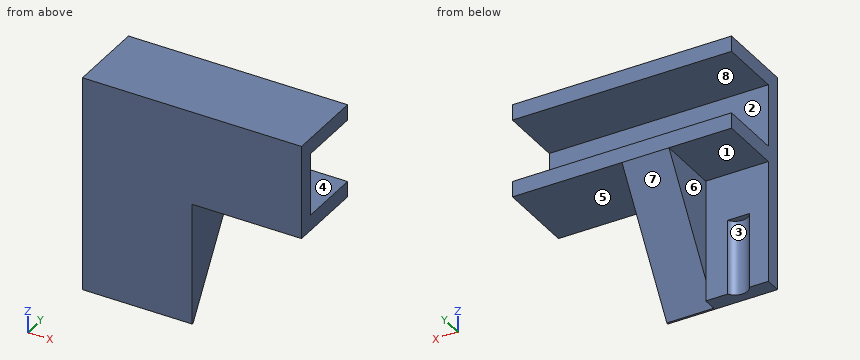
Autodesk Inventor part; units mm, degrees
ref_plane "YZ Plane" through (0, 0, 0) normal (1, 0, 0) x (0, 1, 0)
ref_plane "XZ Plane" through (0, 0, 0) normal (0, 1, 0) x (-1, 0, 0)
ref_plane "XY Plane" through (0, 0, 0) normal (0, 0, 1) x (1, 0, 0)
sketch "Sketch1" plane through (0, 0, 0) normal (0, 1, 0) x (-1, 0, 0)
  line L0 (70, 80) -> (0, 80)
  line L1 (0, 80) -> (0, 0)
  line L2 (0, 0) -> (70, 0)
  line L3 (70, 0) -> (70, 80)
  line L4 (0, 0) -> (30, 0)
  line L5 (30, 0) -> (30, 60)
  line L6 (30, 60) -> (0, 60)
  line L7 (0, 60) -> (0, 0)
  point P0 (0, 60)
  dimension "d0" = 80
  dimension "d1" = 70
  dimension "d2" = 30
  dimension "d3" = 60
extrude "Extrusion1" add sketch "Sketch1" along normal blind 10 contours L3 L2 L5 L6 L1 L0
sketch "Sketch2" plane through (0, 0, 80) normal (1, 0, 0) x (0, 0, -1)
  line L0 (0, 0) -> (20, 0) construction
  line L1 (0, 10) -> (20, 10) construction
  line L2 (0, 0) -> (0, 10) construction
  line L3 (-50, 0) -> (0, 0)
  line L4 (0, 0) -> (0, 50)
  line L5 (0, 50) -> (-10, 50)
  line L6 (-10, 50) -> (-10, 10)
  line L7 (-10, 10) -> (-50, 10)
  line L8 (-50, 10) -> (-50, 0)
  point P0 (80, 0)
  dimension "d6" = 50
  dimension "d7" = 50
  dimension "d8" = 40
  dimension "d9" = 40
extrude "Extrusion2" add sketch "Sketch2" along normal mid plane 140
sketch "Sketch4" plane through (-30, 0, 0) normal (0, 0, -1) x (-1, 0, 0)
  circle A0 centre (21, 14) radius 8.0623
  point P0 (-30, 0)
extrude "Extrusion3" cut sketch "Sketch4" against normal blind 50
sketch "Sketch6" plane through (-30, 0, 60) normal (1, 0, 0) x (0, 0, -1)
  line L0 (-20, 50) -> (-20, 10) construction
  line L1 (60, 0) -> (-20, 50)
  line L2 (-20, 50) -> (-20, 0)
  line L3 (-20, 0) -> (60, 0)
extrude "Extrusion4" add sketch "Sketch6" along normal blind 30
sketch "Sketch7" plane through (-70, 0, 0) normal (-1, 0, 0) x (0, 0, 1)
  line L0 (2, 52) -> (-22, 52)
  line L1 (-22, 52) -> (-22, -1)
  line L2 (-22, -1) -> (2, -1)
  line L3 (2, -1) -> (2, 52)
extrude "Extrusion5" cut sketch "Sketch7" against normal blind 1000
sketch "Sketch8" plane through (-70, 0, 2) normal (-1, 0, 0) x (0, 0, 1)
  line L0 (128, 0) -> (138, 0)
  line L1 (138, 0) -> (138, 50)
  line L2 (138, 50) -> (128, 50)
  line L3 (128, 50) -> (128, 0)
  point P0 (-2, 0)
  dimension "d18" = 10
extrude "Extrusion6" add sketch "Sketch8" against normal up to surface (140 mm away)
properties part number "GiroMotorKrepl"
Design review of the part built by this model. Coordinates are the model's own, in mm. Face numbers are marked on the shaded views. A direction names the side the tool comes from. Round coordinates to 2 decimals unless told otherwise and drop trailing zeros. Write each loop counter-clockwise with the first axis right and the second up, starting at its lowest first coordinate (ties: lowest second). Pieces come first, ordered by that corner, then holes. Notation, with made-up numbers: (47.25, 47) - (95.25, 47) arc R25 ccw to (95.25, 71) - close; hole circle Ø11 at (32, 38). An arc over 180 degrees is marked (long way). Return JSON: item names as keys, results as strings. Group by question number.
Item 1: Machinability: for the marked faces 5, 6, 7 and 8, which of the approach directions +Z, -Z, +X, -X, +Y, -Y give a long, thin tool a straight path to every point of the face, cutting with its end or side? Answer none if there is none.
Item 2: We need section A-A on y = 32.5. Write out the cut boundary in (x, z).
Item 3: Insertion check: P1, Ø25, axis at x = 37, y = 20, coming from the -Z side; P2, Ø12, axis at x = 52.5, z = 122.5, coming from the +Y side; P3, Ø2.5, axis at y = 5, z = 6.5, coming from the +X side. Each pin has a flat end and moves straight along its axis. Give the tip position at first contact, or say it passes through.
Item 4: For probe 1 along Z at (x, y) = (-35.5, 46); probe 2 along X at (y, z) = (24, 41); probe 3 along Y at (x, z) = (-43, 18.5), list the stretches that pass through material, from the lowest coordinate up. Write a range as [from, to].
Item 5: We need section D-D on y = 14. Write out the cut boundary in (x, z).
Item 6: We need section C-C on z = 24. Write out the cut boundary in (x, y), and give its area (3 significant figures).
Item 7: We need section B-B on x = -22.5. Write out the cut boundary in (y, z).
Item 8: The part is to be moulded in two halves that separate along Z. For the marked faces 1, 2, 3 and 4, say which applies: pulls with the +Z half, pulls with the -Z half, needs draft (parallel to the pull), parting line crosses it, or undercut.
Model answer:
{
 "1": {"face 5": "-Z, +X, +Y, -Y", "face 6": "-Z, -X, +Y", "face 7": "-Z, +X, +Y", "face 8": "+X, -X, +Y"},
 "2": {"outline": "(-70, 80) - (-30, 80) - (-30, 52) - (0, 52) - (0, 80) - (70, 80) - (70, 90) - (-70, 90) - close; (-70, 130) - (70, 130) - (70, 140) - (-70, 140) - close"},
 "3": {"P1": "stops at z = 80", "P2": "stops at y = 10", "P3": "stops at x = 0"},
 "4": {"probe 1": "z = [80, 90], [130, 140]", "probe 2": "x = [-30, 0]", "probe 3": "y = [0, 10]"},
 "5": {"outline": "(-70, 80) - (-30, 80) - (-30, 22.4) - (0, 22.4) - (0, 80) - (70, 80) - (70, 90) - (-70, 90) - close; (-70, 130) - (70, 130) - (70, 140) - (-70, 140) - close"},
 "6": {"outline": "(-70, 0) - (0, 0) - (0, 15) - (-30, 15) - (-30, 10) - (-44, 10) arc R8.06 cw to (-58, 10) - (-70, 10) - close", "area": "810 mm²"},
 "7": {"outline": "(0, 2) - (1.25, 2) - (50, 80) - (50, 90) - (10, 90) - (10, 130) - (50, 130) - (50, 140) - (0, 140) - close"},
 "8": {"face 1": "pulls with the -Z half", "face 2": "undercut", "face 3": "needs draft", "face 4": "undercut"}
}
